Build history of the part. All positions in model axes, mm. A direction names the side the tool comes from. Coordinates: 2 decimals unless noted, no trailing zeros. Write each loop counter-clockwise with the first axis right and the second up, starting at its lowest first coordinate (ties: lowest second). Pieces come first, ordered by that corner, then holes. Notation, with made-up numbers: M 85.5,54 L 94.5,54 A21 ccw 94.5,63 Z; hole C 18,78.5 d9. An arc over 180 degrees is marked long. Use CSV: the item, a comma, the result in double quotes. Start each with the question number.
```python
from build123d import *

# Parameters (mm, degrees)
F0_W      = 150
F0_H      = 73
F1_DEPTH  = 7.873
F2_W      = 136
F2_H      = 63
F3_DEPTH  = 4.873
F4_R      = 1.25
F5_DEPTH  = 7.873
F6_R      = 1.25
F7_DEPTH  = 7.873
F8_R      = 1.25
F9_DEPTH  = 7.873
F10_R     = 1.25
F11_DEPTH = 7.873
F12_R     = 1.25
F13_DEPTH = 7.873
F14_R     = 1.25
F15_DEPTH = 7.873
F16_R     = 1.25
F17_DEPTH = 7.873
F18_R     = 1.25
F19_DEPTH = 7.873
F20_R     = 1.25
F21_DEPTH = 7.873
F22_R     = 1.25
F23_DEPTH = 7.873
F24_R     = 1.25
F25_DEPTH = 7.873
F26_R     = 1.25
F27_DEPTH = 7.873
F28_R     = 1.25
F29_DEPTH = 7.873
F30_R     = 1.25
F31_DEPTH = 7.873
F32_R     = 1.25
F33_DEPTH = 7.873
F34_R     = 1.25
F35_DEPTH = 7.873
F36_R     = 1.25
F37_DEPTH = 7.873
F38_R     = 1.25
F39_DEPTH = 7.873
F40_R     = 1.25
F41_DEPTH = 7.873
F42_R     = 1.25
F43_DEPTH = 7.873
F44_R     = 1.25
F45_DEPTH = 7.873
F46_R     = 1.25
F47_DEPTH = 7.873
F48_R     = 1.25
F49_DEPTH = 7.873
F50_R     = 1.25
F51_DEPTH = 7.873
F52_R     = 1.25
F53_DEPTH = 7.873
F54_R     = 1.25
F55_DEPTH = 7.873
F56_R     = 2
F57_DEPTH = 3
F58_R     = 2
F59_DEPTH = 3
F60_R     = 2
F61_DEPTH = 3
F62_R     = 2
F63_DEPTH = 3
F64_R     = 2
F65_DEPTH = 3
F66_R     = 2
F67_DEPTH = 3
F68_R     = 2
F69_DEPTH = 3
F70_R     = 2
F71_DEPTH = 3
F72_R     = 2
F73_DEPTH = 3
F74_R     = 2
F75_DEPTH = 3
F76_W     = 2.5
F76_H     = 4.873
F77_DEPTH = 63
F78_W     = 2.5
F78_H     = 6.5
F79_DEPTH = 0.623
F80_R     = 2
F81_DEPTH = 10
F82_R     = 2
F83_DEPTH = 10
F84_R     = 2
F85_DEPTH = 10
F86_R     = 2
F87_DEPTH = 10
F88_R     = 2
F89_DEPTH = 10
F90_R     = 2
F91_DEPTH = 10


with BuildPart() as f1:
    # F0 (on Top) → F1 (new body)
    with BuildSketch(Plane.XY):
        with Locations((75, 36.5)):
            Rectangle(F0_W, F0_H)
    extrude(amount=F1_DEPTH)

    # F2 (on Top) → F3 (cut)
    with BuildSketch(Plane.XY):
        with Locations((75, 36.5)):
            Rectangle(F2_W, F2_H)
    extrude(amount=F3_DEPTH, mode=Mode.SUBTRACT)

    # F4 (on face) → F5 (cut)
    with BuildSketch(Plane.XY.offset(7.873)):
        with Locations((2.5, 2.5)):
            Circle(F4_R)
    extrude(amount=-F5_DEPTH, mode=Mode.SUBTRACT)

    # F6 (on face) → F7 (cut)
    with BuildSketch(Plane.XY.offset(7.873)):
        with Locations((18, 2.5)):
            Circle(F6_R)
    extrude(amount=-F7_DEPTH, mode=Mode.SUBTRACT)

    # F8 (on face) → F9 (cut)
    with BuildSketch(Plane.XY.offset(7.873)):
        with Locations((34.5, 2.5)):
            Circle(F8_R)
    extrude(amount=-F9_DEPTH, mode=Mode.SUBTRACT)

    # F10 (on face) → F11 (cut)
    with BuildSketch(Plane.XY.offset(7.873)):
        with Locations((51, 2.5)):
            Circle(F10_R)
    extrude(amount=-F11_DEPTH, mode=Mode.SUBTRACT)

    # F12 (on face) → F13 (cut)
    with BuildSketch(Plane.XY.offset(7.873)):
        with Locations((67.5, 2.5)):
            Circle(F12_R)
    extrude(amount=-F13_DEPTH, mode=Mode.SUBTRACT)

    # F14 (on face) → F15 (cut)
    with BuildSketch(Plane.XY.offset(7.873)):
        with Locations((82.5, 2.5)):
            Circle(F14_R)
    extrude(amount=-F15_DEPTH, mode=Mode.SUBTRACT)

    # F16 (on face) → F17 (cut)
    with BuildSketch(Plane.XY.offset(7.873)):
        with Locations((99, 2.5)):
            Circle(F16_R)
    extrude(amount=-F17_DEPTH, mode=Mode.SUBTRACT)

    # F18 (on face) → F19 (cut)
    with BuildSketch(Plane.XY.offset(7.873)):
        with Locations((115.5, 2.5)):
            Circle(F18_R)
    extrude(amount=-F19_DEPTH, mode=Mode.SUBTRACT)

    # F20 (on face) → F21 (cut)
    with BuildSketch(Plane.XY.offset(7.873)):
        with Locations((132, 2.5)):
            Circle(F20_R)
    extrude(amount=-F21_DEPTH, mode=Mode.SUBTRACT)

    # F22 (on face) → F23 (cut)
    with BuildSketch(Plane.XY.offset(7.873)):
        with Locations((147.5, 2.5)):
            Circle(F22_R)
    extrude(amount=-F23_DEPTH, mode=Mode.SUBTRACT)

    # F24 (on face) → F25 (cut)
    with BuildSketch(Plane.XY.offset(7.873)):
        with Locations((2.5, 22)):
            Circle(F24_R)
    extrude(amount=-F25_DEPTH, mode=Mode.SUBTRACT)

    # F26 (on face) → F27 (cut)
    with BuildSketch(Plane.XY.offset(7.873)):
        with Locations((147.5, 22)):
            Circle(F26_R)
    extrude(amount=-F27_DEPTH, mode=Mode.SUBTRACT)

    # F28 (on face) → F29 (cut)
    with BuildSketch(Plane.XY.offset(7.873)):
        with Locations((147.5, 38.5)):
            Circle(F28_R)
    extrude(amount=-F29_DEPTH, mode=Mode.SUBTRACT)

    # F30 (on face) → F31 (cut)
    with BuildSketch(Plane.XY.offset(7.873)):
        with Locations((2.5, 38.5)):
            Circle(F30_R)
    extrude(amount=-F31_DEPTH, mode=Mode.SUBTRACT)

    # F32 (on face) → F33 (cut)
    with BuildSketch(Plane.XY.offset(7.873)):
        with Locations((2.5, 55)):
            Circle(F32_R)
    extrude(amount=-F33_DEPTH, mode=Mode.SUBTRACT)

    # F34 (on face) → F35 (cut)
    with BuildSketch(Plane.XY.offset(7.873)):
        with Locations((147.5, 55)):
            Circle(F34_R)
    extrude(amount=-F35_DEPTH, mode=Mode.SUBTRACT)

    # F36 (on face) → F37 (cut)
    with BuildSketch(Plane.XY.offset(7.873)):
        with Locations((2.5, 70.5)):
            Circle(F36_R)
    extrude(amount=-F37_DEPTH, mode=Mode.SUBTRACT)

    # F38 (on face) → F39 (cut)
    with BuildSketch(Plane.XY.offset(7.873)):
        with Locations((147.5, 70.5)):
            Circle(F38_R)
    extrude(amount=-F39_DEPTH, mode=Mode.SUBTRACT)

    # F40 (on face) → F41 (cut)
    with BuildSketch(Plane.XY.offset(7.873)):
        with Locations((18, 70.5)):
            Circle(F40_R)
    extrude(amount=-F41_DEPTH, mode=Mode.SUBTRACT)

    # F42 (on face) → F43 (cut)
    with BuildSketch(Plane.XY.offset(7.873)):
        with Locations((132, 70.5)):
            Circle(F42_R)
    extrude(amount=-F43_DEPTH, mode=Mode.SUBTRACT)

    # F44 (on face) → F45 (cut)
    with BuildSketch(Plane.XY.offset(7.873)):
        with Locations((34.5, 70.5)):
            Circle(F44_R)
        Circle(F44_R)
    extrude(amount=-F45_DEPTH, mode=Mode.SUBTRACT)

    # F46 (on face) → F47 (cut)
    with BuildSketch(Plane.XY.offset(7.873)):
        with Locations((115.5, 70.5)):
            Circle(F46_R)
    extrude(amount=-F47_DEPTH, mode=Mode.SUBTRACT)

    # F48 (on face) → F49 (cut)
    with BuildSketch(Plane.XY.offset(7.873)):
        with Locations((51, 70.5)):
            Circle(F48_R)
    extrude(amount=-F49_DEPTH, mode=Mode.SUBTRACT)

    # F50 (on face) → F51 (cut)
    with BuildSketch(Plane.XY.offset(7.873)):
        with Locations((67.5, 70.5)):
            Circle(F50_R)
    extrude(amount=-F51_DEPTH, mode=Mode.SUBTRACT)

    # F52 (on face) → F53 (cut)
    with BuildSketch(Plane.XY.offset(7.873)):
        with Locations((82.5, 70.5)):
            Circle(F52_R)
    extrude(amount=-F53_DEPTH, mode=Mode.SUBTRACT)

    # F54 (on face) → F55 (cut)
    with BuildSketch(Plane.XY.offset(7.873)):
        with Locations((99, 70.5)):
            Circle(F54_R)
    extrude(amount=-F55_DEPTH, mode=Mode.SUBTRACT)

    # F56 (on face) → F57 (cut)
    with BuildSketch(Plane.XY.offset(7.873)):
        with Locations((41, 64.1)):
            Circle(F56_R)
    extrude(amount=-F57_DEPTH, mode=Mode.SUBTRACT)

    # F58 (on face) → F59 (cut)
    with BuildSketch(Plane.XY.offset(7.873)):
        with Locations((41, 58.3)):
            Circle(F58_R)
    extrude(amount=-F59_DEPTH, mode=Mode.SUBTRACT)

    # F60 (on face) → F61 (cut)
    with BuildSketch(Plane.XY.offset(7.873)):
        with Locations((19.15, 36.5)):
            Circle(F60_R)
    extrude(amount=-F61_DEPTH, mode=Mode.SUBTRACT)

    # F62 (on face) → F63 (cut)
    with BuildSketch(Plane.XY.offset(7.873)):
        with Locations((68.6, 36.5)):
            Circle(F62_R)
    extrude(amount=-F63_DEPTH, mode=Mode.SUBTRACT)

    # F64 (on face) → F65 (cut)
    with BuildSketch(Plane.XY.offset(7.873)):
        with Locations((109, 64.1)):
            Circle(F64_R)
    extrude(amount=-F65_DEPTH, mode=Mode.SUBTRACT)

    # F66 (on face) → F67 (cut)
    with BuildSketch(Plane.XY.offset(7.873)):
        with Locations((109, 58.3)):
            Circle(F66_R)
    extrude(amount=-F67_DEPTH, mode=Mode.SUBTRACT)

    # F68 (on face) → F69 (cut)
    with BuildSketch(Plane.XY.offset(7.873)):
        with Locations((81.4, 36.5)):
            Circle(F68_R)
    extrude(amount=-F69_DEPTH, mode=Mode.SUBTRACT)

    # F70 (on face) → F71 (cut)
    with BuildSketch(Plane.XY.offset(7.873)):
        with Locations((130.85, 36.5)):
            Circle(F70_R)
    extrude(amount=-F71_DEPTH, mode=Mode.SUBTRACT)

    # F72 (on face) → F73 (cut)
    with BuildSketch(Plane.XY.offset(7.873)):
        with Locations((58, 20)):
            Circle(F72_R)
    extrude(amount=-F73_DEPTH, mode=Mode.SUBTRACT)

    # F74 (on face) → F75 (cut)
    with BuildSketch(Plane.XY.offset(7.873)):
        with Locations((92, 20)):
            Circle(F74_R)
    extrude(amount=-F75_DEPTH, mode=Mode.SUBTRACT)

    # F76 (on face) → F77 (join)
    with BuildSketch(Plane(origin=(0, 5, 0), x_dir=(-1, 0, 0), z_dir=(0, 1, 0))):
        with Locations((-75, 2.4365)):
            Rectangle(F76_W, F76_H)
    extrude(amount=F77_DEPTH)

    # F78 (on face) → F79 (cut)
    with BuildSketch(Plane(origin=(0, 0, 0), x_dir=(1, 0, 0), z_dir=(0, 0, -1))):
        with Locations((75, -36.5)):
            Rectangle(F78_W, F78_H)
    extrude(amount=-F79_DEPTH, mode=Mode.SUBTRACT)

    # F80 (on face) → F81 (join)
    with BuildSketch(Plane(origin=(0, 0, 4.873), x_dir=(1, 0, 0), z_dir=(0, 0, -1))):
        with Locations((41, -14.7)):
            Circle(F80_R)
    extrude(amount=F81_DEPTH)

    # F82 (on face) → F83 (join)
    with BuildSketch(Plane(origin=(0, 0, 4.873), x_dir=(1, 0, 0), z_dir=(0, 0, -1))):
        with Locations((41, -36.5)):
            Circle(F82_R)
    extrude(amount=F83_DEPTH)

    # F84 (on face) → F85 (join)
    with BuildSketch(Plane(origin=(0, 0, 4.873), x_dir=(1, 0, 0), z_dir=(0, 0, -1))):
        with Locations((109, -36.5)):
            Circle(F84_R)
    extrude(amount=F85_DEPTH)

    # F86 (on face) → F87 (join)
    with BuildSketch(Plane(origin=(0, 0, 4.873), x_dir=(1, 0, 0), z_dir=(0, 0, -1))):
        with Locations((109, -14.7)):
            Circle(F86_R)
    extrude(amount=F87_DEPTH)

    # F88 (on face) → F89 (join)
    with BuildSketch(Plane(origin=(0, 0, 4.873), x_dir=(1, 0, 0), z_dir=(0, 0, -1))):
        with Locations((61.55, -36.5)):
            Circle(F88_R)
    extrude(amount=F89_DEPTH)

    # F90 (on face) → F91 (join)
    with BuildSketch(Plane(origin=(0, 0, 4.873), x_dir=(1, 0, 0), z_dir=(0, 0, -1))):
        with Locations((88.45, -36.5)):
            Circle(F90_R)
    extrude(amount=F91_DEPTH)


solid = f1.part
```
1. Slice it at C-C (x = 136). List the corners of the cut face in (y, z), and give its area (3 significant figures).
2. 3-axis set-ups, long thin cutter, end or side, ignore diameter. For faces 4 (the flat face through (74, 37, 7.873)), 5 (the flat face through (76.25, 36, 2)): which of +Z, -Z, +X, -X, +Y, -Y reach the whole face in a straight line?
3. Slice it at D-D (y = 26). List the corners of the cut face in (x, z).
4. Drill centre lines: line 1 along Y through (x, z) = (82.5, 2); line 2 along X through (y, z) = (59.5, 1); line 3 along Y through (x, z) = (109, 7.25). Where is each one in solid material? Low to high. Write a range as from..to.
5. Slice it at B-B (z = 2.5). Count the separate pieces of the cut face and the enclosed holes in it, and give its area (3 significant figures).
6. Slice it at A-A (y = 64.1). List the corners of the cut face in (x, z).
7. Pull direction X, two halves, no side cores. Call faces 1 (the flat face through (109, 15, -5.127)), 2 (the cylindrical face through (93.908, 20.601, 6.394)), 3 (the flat face through (0, 37, 4)): pulls with the +X half, pulls with the -X half, needs draft (parallel to the pull), parting line crosses it, or undercut.
8. Flat gauge pins, fed straight in: pin 1 (5 mm diameter, centred on x = 125.5, y = 19, fed in from -Z); pin 2 (2 mm diameter, centred on x = 34.5, y = 2.5, fed in from +Z); pin 3 (4 mm diameter, centred on x = 82.5, y = 70.5, fed in from -Z). Where does each tip first touch, or does it go through?
Established:
1,outline,"M 0,0 L 5,0 L 5,4.87 L 68,4.87 L 68,0 L 73,0 L 73,7.87 L 0,7.87 Z"
1,area,"268 mm2"
2,face 4,"+Z, +X, -X, +Y, -Y"
2,face 5,"-Z"
3,outline,"M 0,0 L 7,0 L 7,4.87 L 73.75,4.87 L 73.75,0 L 76.25,0 L 76.25,4.87 L 143,4.87 L 143,0 L 150,0 L 150,7.87 L 0,7.87 Z"
4,line 1,"y = 0..1.25, 3.75..5, 68..69.25, 71.75..73"
4,line 2,"x = 0..7, 73.75..76.25, 143..150"
4,line 3,"y = 0..56.3, 60.3..62.1, 66.1..73"
5,separate pieces,"7"
5,enclosed holes,"28"
5,area,"2,490 mm2"
6,outline,"M 0,0 L 7,0 L 7,4.87 L 39,4.87 L 39,7.87 L 0,7.87 Z; M 43,4.87 L 73.75,4.87 L 73.75,0 L 76.25,0 L 76.25,4.87 L 107,4.87 L 107,7.87 L 43,7.87 Z; M 111,4.87 L 143,4.87 L 143,0 L 150,0 L 150,7.87 L 111,7.87 Z"
7,face 1,"needs draft"
7,face 2,"undercut"
7,face 3,"pulls with the -X half"
8,pin 1,"stops at z = 4.87"
8,pin 2,"passes through"
8,pin 3,"stops at z = 0"
